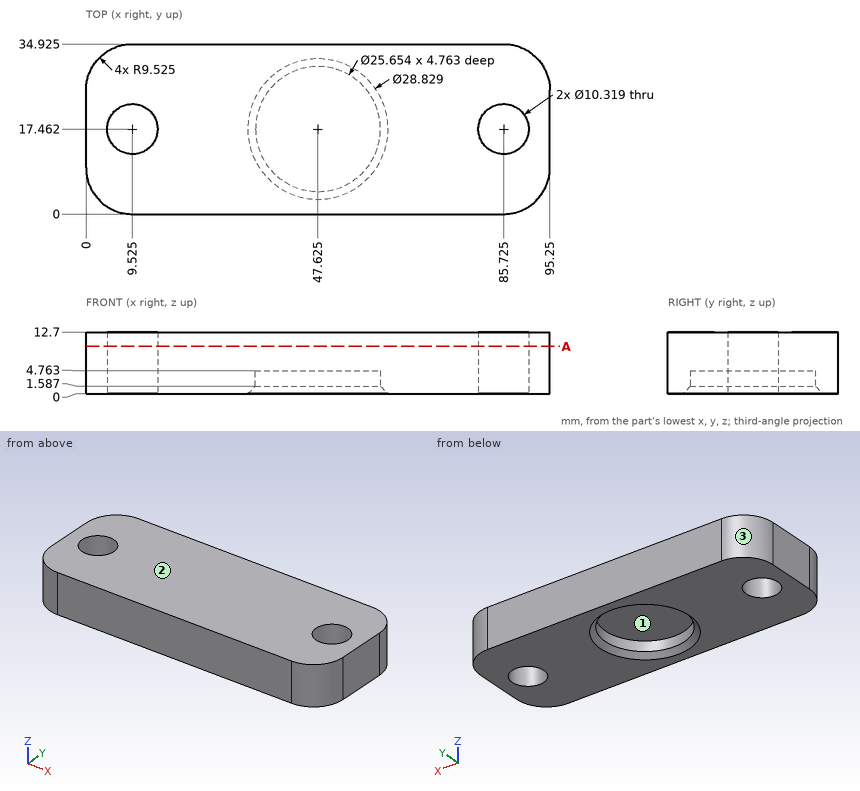
Answer from the drawing. Dimensions are ordinates in mm from the lowest x, y and z of the part. Round coordinates to 2 decimals unless told otherwise and drop trailing zeros.
1) Consider line 1 (Y direction, x = 86, z = 4.25) (1 decimal); line 2 (X direction, y = 15, z = 8.25); line 3 (Z direction, x = 54.5, y = 19). Determine where each line is inside the solid, lowest interval first.
Outcome:
line 1: y = 0 to 12.3, 22.6 to 34.9
line 2: x = 0 to 4.99, 14.06 to 81.19, 90.26 to 95.25
line 3: z = 4.76 to 12.7
2) A cutting plane is placed at A-A on z = 9.75. Give the number of separate pieces and of enclosed holes in the cut face, plus the area to 3 significant figures.
Outcome:
separate pieces: 1
enclosed holes: 2
area: 3,080 mm2
3) For a pull along Y with two mould halves and no side action, classify the marked faces 1, 2 and 3 as released by +Y, released by -Y, zero draft, split by the parting line, or undercut.
Outcome:
face 1: undercut
face 2: zero draft
face 3: released by +Y
4) Given P1, Ø7.5, axis at x = 41.5, y = 16.5, coming from the -Z side; P2, Ø6, axis at x = 85.72, y = 17.46, coming from the -Z side, each flat-ended and moving along its own axis, determine where each tip first touches the part or whether it passes through.
Outcome:
P1: stops at z = 4.76
P2: passes through
